Source: CAD feature listing. Evaluate the final solid. Frame: model axes, mm. Face numbers are marked on the shaded views. A direction names the side the tool comes from. Give positions to 0.01 mm unless a question says otherwise; leave off trailing zeros. Loops run counter-clockwise (first coordinate to the right, second up) from the corner with the lowest first, then second, coordinate; pieces in that order, holes last. Notation, with made-up numbers: (3, 60.25) -> (20, 60.25) arc R14 cw to (20, 87.25) -> close; hole circle Ø1 at (64, 83). An arc over 180 degrees is marked (long way). Return JSON: item names as keys, results as strings. Group by question number.
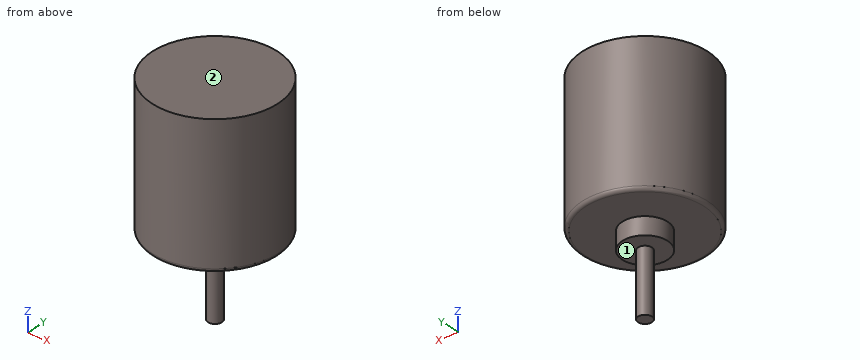
```python
from build123d import *

# Parameters (mm, degrees)
F0_R     = 18
F1_DEPTH = 40
F2_R     = 6.5
F3_DEPTH = 5
F4_R     = 2
F5_DEPTH = 23
F6_R     = 1


with BuildPart() as f1:
    # F0 (on Top) → F1 (new body)
    with BuildSketch(Plane.XY):
        Circle(F0_R)
    extrude(amount=F1_DEPTH)

    # F2 (on Top) → F3 (join)
    with BuildSketch(Plane.XY):
        Circle(F2_R)
    extrude(amount=-F3_DEPTH)

    # F4 (on Top) → F5 (join)
    with BuildSketch(Plane.XY):
        Circle(F4_R)
    extrude(amount=-F5_DEPTH)

    # F6
    f6_edges = [f1.edges().sort_by_distance(p)[0] for p in [
        (-18, 0, 0),
    ]]
    fillet(f6_edges, radius=F6_R)


solid = f1.part
```
1) Cut plane C-C on z = -9. Return loops of the section in (x, y), then the cut area to 3 significant figures.
2) Contact query for flat-ended pins moving along their axis: P1, Ø8, axis at y = 9, z = 3.5, coming from the -X side; P2, Ø6, axis at x = -13, z = 26.5, coming from the +Y side; P3, Ø1.5, axis at y = -2, z = 9.5, coming from the +X side. Output: stop coordinate, or through.
3) Material intervals for line 1 (Z direction, x = 11, y = 7); line 2 (X direction, y = 0.5, z = 33.5); line 3 (Z direction, x = 2, y = -3.5), sorted ascending.
4) Reachability of the marked faces 1 and 2 from +Z, -Z, +X, -X, +Y, -Y: full face, straight path, thin tool, end or side. Return the list, or none.
5) Cut plane A-A on x = 0. Return loops of the section in (y, z), then the cut area to 3 significant figures.
Calculated:
{
 "1": {"outline": "circle Ø4 at (0, 0)", "area": "12.6 mm2"},
 "2": {"P1": "x = -17.29", "P2": "y = 14.97", "P3": "x = 17.96"},
 "3": {"line 1": "0 to 40", "line 2": "-17.99 to 17.99", "line 3": "-5 to 40"},
 "4": {"face 1": "-Z", "face 2": "+Z, +X, -X, +Y, -Y"},
 "5": {"outline": "(-18, 1) arc R1 ccw to (-17, 0) -> (-6.5, 0) -> (-6.5, -5) -> (-2, -5) -> (-2, -23) -> (2, -23) -> (2, -5) -> (6.5, -5) -> (6.5, 0) -> (17, 0) arc R1 ccw to (18, 1) -> (18, 40) -> (-18, 40) -> close", "area": "1,580 mm2"}
}
